Check sheet for the drawn part. Datum: minimum x, y, z corner. Units: mm. Coordinates: 2 decimals unless noted, no trailing zeros. Loops run counter-clockwise (first coordinate to the right, second up) from the corner with the lowest first, then second, coordinate; pieces in that order, holes last. Notation, with made-up numbers: M 49,24.5 L 86,24.5 A27 ccw 86,46.5 Z; hole C 27.25,-36.5 d8. An arc over 180 degrees is marked long. Use CSV: the item, a comma, the result in double quotes. Start each with the question number.
(1) Scan lines: line 1 (X direction, y = 21.5, z = 7.5); line 2 (X direction, y = 28, z = 8.25); line 3 (Z direction, x = 7.5, y = 21.5). Record each from-to range of solid material in increasing order.
(2) Section check A-A on y = 24.5. Record the cut outline in (x, z) (1 decimal), and give its area (3 significant figures).
(3) Draft check along X on the marked faces 1, 2 and 3. Enter one of: pulls with the +X half, pulls with the -X half, needs draft (parallel to the pull), parting line crosses it, or undercut.
(4) Section check C-C on y = 16.5. Record the cut outline in (x, z), and give its area (3 significant figures).
(5) Section check D-D on z = 13.25. Record the cut outline in (x, y), and give its area (3 significant figures).
(6) Section check B-B on x = 12. Record the cut outline in (y, z), and give its area (3 significant figures).
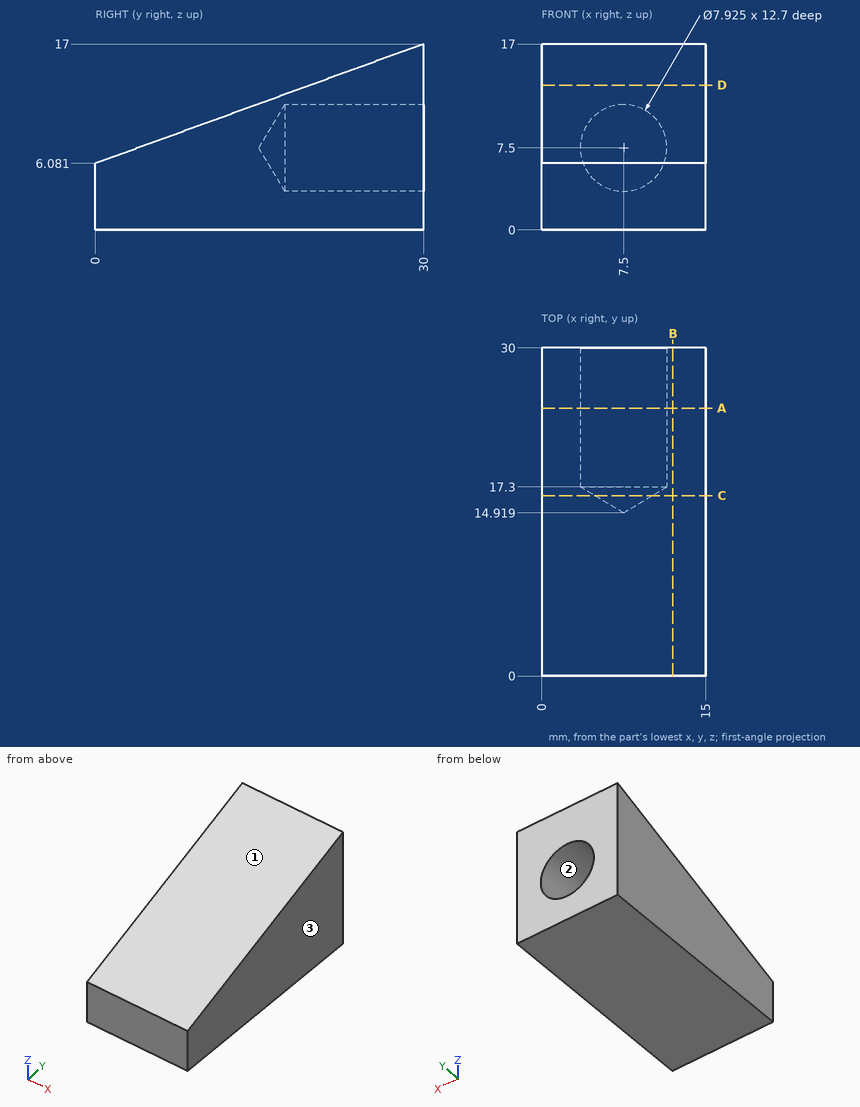
Outcome:
1,line 1,"x = 0 to 3.54, 11.46 to 15"
1,line 2,"x = 0 to 3.61, 11.39 to 15"
1,line 3,"z = 0 to 3.54, 11.46 to 13.91"
2,outline,"M 0,0 L 15,0 L 15,15 L 0,15 Z; hole C 7.5,7.5 d7.9"
2,area,"176 mm²"
3,face 1,"needs draft"
3,face 2,"undercut"
3,face 3,"pulls with the +X half"
4,outline,"M 0,0 L 15,0 L 15,12.09 L 0,12.09 Z; hole C 7.5,7.5 d5.26"
4,area,"160 mm²"
5,outline,"M 0,19.7 L 15,19.7 L 15,30 L 0,30 Z"
5,area,"155 mm²"
6,outline,"M 0,0 L 30,0 L 30,17 L 0,6.08 Z"
6,area,"346 mm²"
